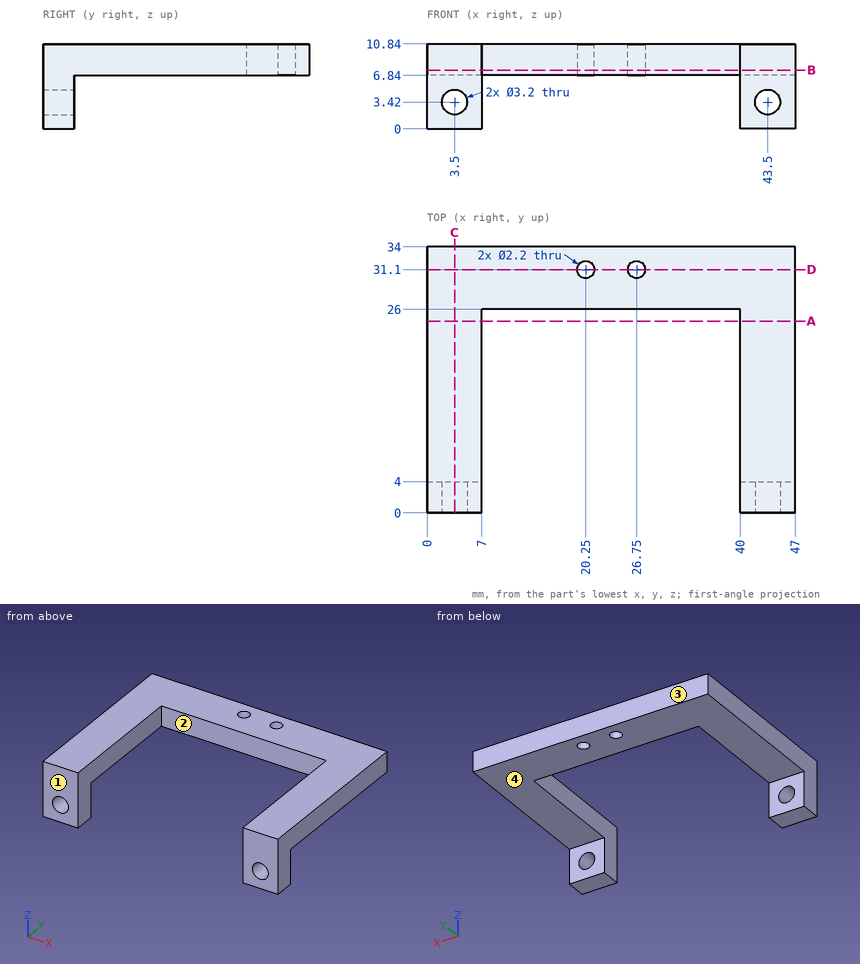
Study the drawing (mm; zero at the part's minimum x, y, z) and answer. A direction names the side the tool comes from. Round coordinates to 2 decimals unless told otherwise and drop trailing zeros. Order: outer loops, then holes, each group sorted by start corner. A loop starts at its lowest first (then second) coordinate and runs counter-clockwise, first axis right, second up. Notation, with made-up numbers: (-10, 3.5) -> (32, 3.5) arc R34 cw to (32, 38.5) -> close; hole circle Ø1 at (14.25, 68). An arc over 180 degrees is marked (long way). Answer as CSV lines item,"result". Start each with the question number.
(1) Find the intervals of material crossed by probe 1 along X at (y, z) = (19, 9.75); probe 2 along Z at (x, y) = (43.5, 0.9); probe 3 along Z at (x, y) = (10, 31), in increasing order. Write a range as from..to.
(2) The part is cut by section D-D (y = 31.1). Determine the outline of the cut face in (x, z).
(3) For a pull along X with two mould halves and no side action, classify the marked faces 1 and 2 as +X half, -X half, draft (parallel to the pull), parting line (faces both ways), or undercut.
(4) A tool of negligible diameter and unlimited length cuts with its end or side. For the marked faces 3 and 4, from which of +Z, -Z, +X, -X, +Y, -Y can it reach the whole face along a straight path? Write none if from no direction.
(5) The part is cut by section C-C (x = 3.5). Determine the outline of the cut face in (y, z), then the cut area to 3 significant figures.
(6) Flat-ended cylindrical pins translate along their axes: pin 1 Ø2.5 at (x, y) = (20.25, 31.1) entering from -Z; pin 2 Ø3.5 at (x, z) = (5, 2.5) entering from +Y; pin 3 Ø3 at (x, z) = (26, 9) entering from -Y. Find the tip coordinate at first contact, or state that the pin passes through.
(7) The part is cut by section A-A (y = 24.5). Determine the outline of the cut face in (x, z), then the cut area to 3 significant figures.
(8) The part is cut by section B-B (z = 7.5). Determine the outline of the cut face in (x, y).
Evaluation:
1,probe 1,"0..7, 40..47"
1,probe 2,"0..1.82, 5.02..10.84"
1,probe 3,"6.84..10.84"
2,outline,"(0, 6.84) -> (19.15, 6.84) -> (19.15, 10.84) -> (0, 10.84) -> close; (21.35, 6.84) -> (25.65, 6.84) -> (25.65, 10.84) -> (21.35, 10.84) -> close; (27.85, 6.84) -> (47, 6.84) -> (47, 10.84) -> (27.85, 10.84) -> close"
3,face 1,"draft"
3,face 2,"undercut"
4,face 3,"+Z, -Z, +X, -X, +Y"
4,face 4,"-Z, +X, -X, +Y"
5,outline,"(0, 0) -> (4, 0) -> (4, 1.82) -> (0, 1.82) -> close; (0, 5.02) -> (4, 5.02) -> (4, 6.84) -> (34, 6.84) -> (34, 10.84) -> (0, 10.84) -> close"
5,area,"151 mm²"
6,pin 1,"z = 6.84"
6,pin 2,"y = 4"
6,pin 3,"y = 26"
7,outline,"(0, 6.84) -> (7, 6.84) -> (7, 10.84) -> (0, 10.84) -> close; (40, 6.84) -> (47, 6.84) -> (47, 10.84) -> (40, 10.84) -> close"
7,area,"56.0 mm²"
8,outline,"(0, 0) -> (7, 0) -> (7, 26) -> (40, 26) -> (40, 0) -> (47, 0) -> (47, 34) -> (0, 34) -> close; hole circle Ø2.2 at (20.25, 31.1); hole circle Ø2.2 at (26.75, 31.1)"
